Autodesk Inventor part; units mm, degrees
ref_plane "YZ Plane" through (0, 0, 0) normal (1, 0, 0) x (0, 1, 0)
ref_plane "XZ Plane" through (0, 0, 0) normal (0, 1, 0) x (-1, 0, 0)
ref_plane "XY Plane" through (0, 0, 0) normal (0, 0, 1) x (1, 0, 0)
sketch "Esquisse3" plane through (0, 0, 0) normal (0, 1, 0) x (-1, 0, 0)
  line L0 (-6.5, 6.5) -> (6.5, 6.5) construction
  line L1 (6.5, 6.5) -> (6.5, -6.5) construction
  line L2 (6.5, -6.5) -> (-6.5, -6.5) construction
  line L3 (-6.5, -6.5) -> (-6.5, 6.5) construction
  line L4 (-6.5, 6.5) -> (6.5, -6.5) construction
  line L5 (6.5, 6.5) -> (-6.5, -6.5) construction
  line L6 (-11.5, 11.5) -> (11.5, 11.5) construction
  line L7 (11.5, 11.5) -> (11.5, -11.5) construction
  line L8 (11.5, -11.5) -> (-11.5, -11.5) construction
  line L9 (-11.5, -11.5) -> (-11.5, 11.5) construction
  line L10 (-11.5, 11.5) -> (11.5, -11.5) construction
  line L11 (11.5, 11.5) -> (-11.5, -11.5) construction
  line L12 (-6.5, 6.5) -> (-11.5, 6.5) construction
  line L13 (-11.5, 6.5) -> (-11.5, 11.5) construction
  line L14 (-11.5, 11.5) -> (-6.5, 11.5) construction
  line L15 (-6.5, 11.5) -> (-6.5, 6.5) construction
  line L16 (-6.5, -6.5) -> (-11.5, -6.5) construction
  line L17 (-11.5, -6.5) -> (-11.5, -11.5) construction
  line L18 (-11.5, -11.5) -> (-6.5, -11.5) construction
  line L19 (-6.5, -11.5) -> (-6.5, -6.5) construction
  line L20 (6.5, -6.5) -> (11.5, -6.5) construction
  line L21 (11.5, -6.5) -> (11.5, -11.5) construction
  line L22 (11.5, -11.5) -> (6.5, -11.5) construction
  line L23 (6.5, -11.5) -> (6.5, -6.5) construction
  line L24 (11.5, 11.5) -> (6.5, 11.5) construction
  line L25 (6.5, 11.5) -> (6.5, 6.5) construction
  line L26 (6.5, 6.5) -> (11.5, 6.5) construction
  line L27 (11.5, 6.5) -> (11.5, 11.5) construction
  circle A0 centre (9, 9) radius 2.5
  circle A1 centre (9, -9) radius 2.5
  circle A2 centre (-9, -9) radius 2.5
  circle A3 centre (-9, 9) radius 2.5
  circle A4 centre (0, 0) radius 17.5
  circle A5 centre (0, 0) radius 8.5
  line L28 (17.5, 0) -> (17.5, 65)
  line L29 (-17.5, 0) -> (-17.5, 65)
  line L30 (0, -17.5) -> (0, 82.5) construction
  circle A6 centre (0, 65) radius 17.5
  circle A7 centre (0, 65) radius 7.5
  line L31 (1.5, 72.3485) -> (-1.5, 72.3485)
  line L32 (-1.5, 72.3485) -> (-1.5, 97.3485)
  line L33 (-1.5, 97.3485) -> (1.5, 97.3485)
  line L34 (1.5, 97.3485) -> (1.5, 72.3485)
  line L35 (-2.5, 98.3485) -> (-2.5, 71.3485)
  line L36 (-2.5, 71.3485) -> (2.5, 71.3485)
  line L37 (2.5, 71.3485) -> (2.5, 98.3485)
  line L38 (2.5, 98.3485) -> (-2.5, 98.3485)
  line L39 (17.5, 63.5) -> (7.3485, 63.5)
  line L40 (7.3485, 63.5) -> (7.3485, 66.5)
  line L41 (7.3485, 66.5) -> (17.5, 66.5)
  line L42 (17.5, 66.5) -> (17.5, 63.5)
  point P0 (17.4356, 66.5)
  point P1 (2.5, 82.3205)
  point P2 (-2.5, 82.3205)
  dimension "d1" = 13
  dimension "d2" = 13
  dimension "d3" = 5
  dimension "d4" = 35
  dimension "d9" = 9
  dimension "d29" = 100
  dimension "d31" = 35
  dimension "d32" = 15
  dimension "d33" = 3
  dimension "d34" = 25
  dimension "d36" = 1
  dimension "d37" = 3
extrude "Extrusion1" add sketch "Esquisse3" along normal blind 2 contours A4 | A4 L29 A6 L39 L28 | A6 L35 A7 L39 | L35 L38 L37 A6 L34 L33 L32 | A6 L32 A7 L35 | L41 A7 L37 A6 | L37 A7 L34 A6
sketch "Esquisse4" plane through (0, 2, 0) normal (0, 1, 0) x (-1, 0, 0)
  circle A0 centre (9, -9) radius 3.5
  circle A1 centre (9, -9) radius 2.5
  circle A2 centre (-9, -9) radius 3.5
  circle A3 centre (-9, 9) radius 3.5
  circle A4 centre (9, 9) radius 3.5
  circle A5 centre (-9, -9) radius 2.5
  circle A6 centre (-9, 9) radius 2.5
  circle A7 centre (9, 9) radius 2.5
  circle A8 centre (0, 0) radius 17.5
  circle A9 centre (0, 0) radius 8.544
  circle A10 centre (-9, -9) radius 2.5
  circle A11 centre (-9, -9) radius 2.5
  circle A12 centre (-9, 9) radius 2.5
  circle A13 centre (9, 9) radius 2.5
  dimension "d10" = 7
  dimension "d11" = 7
  dimension "d12" = 7
  dimension "d13" = 7
extrude "Extrusion2" add sketch "Esquisse4" along normal blind 2 contours A0 | A2 | A3 | A4 | A8
chamfer "Chanfrein1" distance 1 distance2 2 1 edges at (-6.5, 4, -9) measured on face at (-3.3085, 4, -12.0053)
chamfer "Chanfrein2" distance 1 distance2 2 1 edges at (11.5, 4, -9) measured on face at (3.3085, 4, 12.0053)
chamfer "Chanfrein3" distance 1 distance2 2 1 edges at (-6.5, 4, 9) measured on face at (3.3085, 4, 12.0053)
chamfer "Chanfrein4" distance 1 distance2 2 1 edges at (11.5, 4, 9) measured on face at (3.3085, 4, 12.0053)
sketch "Esquisse7" plane through (0, 2, 0) normal (0, 1, 0) x (1, 0, 0)
  point P0 (0, 0)
properties part number "Pièce_moteur_maintient_test_3"
For this review, take the finished solid that the model builds, in its own axes (mm). A direction names the side the tool comes from. Coordinates: 2 decimals unless noted, no trailing zeros. Order: outer loops, then holes, each group sorted by start corner. A loop starts at its lowest first (then second) coordinate and runs counter-clockwise, first axis right, second up. Notation, with made-up numbers: (41, 64.5) -> (45, 64.5) arc R10 cw to (45, 75.5) -> close; hole circle Ø3 at (-36.75, -6). An arc over 180 degrees is marked (long way). Answer as CSV lines item,"result".
Q1. For faces 4 (the face through (2.5, 1, 90)), 5 (the face through (-12, 1, 63.5)), 6 (the face through (4, 4, -8)), 7 (the face through (-5.26, 0.986, 70.346)), list the 3-axis set-ups (+Z, -Z, +X, -X, +Y, -Y) from which the entire face can be reached by the end or side of a thin tool; tool diameter is ignored.
Model answer:
face 4,"+Z, +X, +Y, -Y"
face 5,"-X, +Y, -Y"
face 6,"+Z, -Z, +X, -X, +Y"
face 7,"+Y, -Y"
Q2. We need section C-C (x = -14.5). State the section outline as (y, z) points, plus the area to 3 significant figures.
Model answer:
outline,"(0, -9.8) -> (4, -9.8) -> (4, 9.8) -> (2, 9.8) -> (2, 63.5) -> (0, 63.5) -> close; (0, 66.5) -> (2, 66.5) -> (2, 74.8) -> (0, 74.8) -> close"
area,"202 mm2"
Q3. Clearance check with flat-ended pins moving along their axes: pin 1 Ø8 at (x, z) = (-0.5, 64.5) entering from -Y (3 decimals); pin 2 Ø1 at (x, y) = (11.5, 1.5) entering from -Z; pin 3 Ø1.6 at (x, y) = (-10.5, 1) entering from -Z; pin 4 Ø1 at (x, y) = (6.5, 1.5) entering from -Z. State where each tip first meets the part, or that it passes through.
Model answer:
pin 1,"passes through"
pin 2,"stops at z = -13.61"
pin 3,"stops at z = -14.57"
pin 4,"stops at z = -16.44"
Q4. We need section A-A (x = 0). State the section outline as (y, z) points, plus the area to 3 significant figures.
Model answer:
outline,"(0, -17.5) -> (4, -17.5) -> (4, -8.54) -> (2, -8.54) -> (2, -8.5) -> (0, -8.5) -> close; (0, 8.5) -> (2, 8.5) -> (2, 8.54) -> (4, 8.54) -> (4, 17.5) -> (2, 17.5) -> (2, 57.5) -> (0, 57.5) -> close; (0, 97.35) -> (2, 97.35) -> (2, 98.35) -> (0, 98.35) -> close"
area,"154 mm2"
Q5. We need section B-B (y = 2.6). State the section outline as (x, z) points, plus the area to 3 significant figures.
Model answer:
outline,"circle Ø35 at (0, 0); hole circle Ø5.6 at (-9, -9); hole circle Ø5.6 at (-9, 9); hole circle Ø17.09 at (0, 0); hole circle Ø5.6 at (9, -9); hole circle Ø5.6 at (9, 9)"
area,"634 mm2"
Q6. Wall thickness on line 1 along Z through (x, y) = (0, 1.25); line 2 along Z through (x, y) = (-9.5, 2.6) (3 decimals); line 3 along X through (y, z) = (2.95, -3.5): over which ranges is each line inside the solid? List them lowest first. Write a range as [from, to].
Model answer:
line 1,"z = [-17.5, -8.5], [8.5, 57.5], [97.35, 98.35]"
line 2,"z = [-14.697, -11.755], [-6.245, 6.245], [11.755, 14.697]"
line 3,"x = [-17.15, -7.79], [7.79, 17.15]"
Q7. We need section D-D (z = 78). State the section outline as (x, y) points, plus the area to 3 significant figures.
Model answer:
outline,"(-11.72, 0) -> (-1.5, 0) -> (-1.5, 2) -> (-11.72, 2) -> close; (1.5, 0) -> (11.72, 0) -> (11.72, 2) -> (1.5, 2) -> close"
area,"40.9 mm2"
Q8. Draft analysis for pull direction X (two halves, no side actions). For faces 1 (the face through (0, 1, 97.348)), 2 (the face through (-12, 1, 66.5)), 3 (the face through (2.28, 2.42, -17.35)), state which applies: released by +X, released by -X, zero draft, split by the parting line, or undercut.
Model answer:
face 1,"undercut"
face 2,"zero draft"
face 3,"split by the parting line"
